Verification items for the finished model (mm, model axes). Face numbers are marked on the shaded views. Coordinates: 2 decimals unless noted, no trailing zeros. Loops run counter-clockwise (first coordinate to the right, second up) from the corner with the lowest first, then second, coordinate; pieces in that order, holes last.
Q1. Material ranges on probe 1 along X at (y, z) = (12.5, -59.69); probe 2 along Z at (x, y) = (-127, 17.5); probe 3 along Z at (x, y) = (-137, 17.5), recorded low to high.
Q2. Sectioned sample at A-A (x = -127). Enter the section's corners in (y, z).
Q3. Mould release check, pull along Z, two halves, no side actions. Record for the marked faces 1, 2 and 3: +Z half, -Z half, draft (parallel to the pull), parting line (faces both ways), or undercut.
Q4. Sectioned sample at D-D (z = -141). Enter the section's corners in (x, y).
Q5. Sectioned sample at C-C (y = 8.5). Enter the section's corners in (x, z), then the cut area to 3 significant figures.
Q6. Go/stop test with flat-tipped pins: P1, Ø1, axis at x = -216, y = 13.5, coming from the -Z side; P2, Ø1, axis at y = 13, z = -130.5, coming from the +X side; P3, Ø8, axis at x = -60.5, y = 13.5, coming from the +Z side. Record where each tip stops, or that it passes through.
Q7. Sectioned sample at B-B (z = -59.69). Enter the section's corners in (x, y), then the cut area to 3 significant figures.
Autodesk Inventor part; units mm, degrees
ref_plane "YZ Plane" through (0, 0, 0) normal (1, 0, 0) x (0, 1, 0)
ref_plane "XZ Plane" through (0, 0, 0) normal (0, 1, 0) x (-1, 0, 0)
ref_plane "XY Plane" through (0, 0, 0) normal (0, 0, 1) x (1, 0, 0)
sketch "Sketch1" plane through (0, 0, 0) normal (0, 1, 0) x (-1, 0, 0)
  line L0 (0, 0) -> (254, 0)
  line L1 (254, 0) -> (254, -119.38)
  line L2 (254, -119.38) -> (0, -119.38)
  line L3 (0, -119.38) -> (0, 0)
  line L4 (186.69, 67.31) -> (67.31, 67.31)
  line L5 (67.31, 67.31) -> (67.31, -186.69)
  line L6 (67.31, -186.69) -> (186.69, -186.69)
  line L7 (186.69, -186.69) -> (186.69, 67.31)
  line L8 (186.69, 67.31) -> (254, 0)
  line L9 (67.31, 67.31) -> (0, 0)
  line L10 (186.69, -186.69) -> (254, -119.38)
  line L11 (0, -119.38) -> (67.31, -186.69)
  line L12 (62.2907, -7.1202) -> (161.0967, -7.1202)
  line L13 (164.2717, -10.2952) -> (164.2717, -109.1012)
  line L14 (161.0967, -112.2762) -> (62.2907, -112.2762)
  line L15 (59.1157, -109.1012) -> (59.1157, -10.2952)
  arc A0 (62.2907, -7.1202) -> (59.1157, -10.2952) centre (62.2907, -10.2952) ccw
  arc A1 (164.2717, -10.2952) -> (161.0967, -7.1202) centre (161.0967, -10.2952) ccw
  arc A2 (161.0967, -112.2762) -> (164.2717, -109.1012) centre (161.0967, -109.1012) ccw
  arc A3 (59.1157, -109.1012) -> (62.2907, -112.2762) centre (62.2907, -109.1012) ccw
  point P0 (164.2717, -112.2762)
  point P1 (164.2717, -7.1202)
  point P2 (59.1157, -112.2762)
  dimension "d0" = 254
  dimension "d1" = 119.38
  dimension "d2" = 119.38
  dimension "d3" = 254
  dimension "d8" = 95.1907
  dimension "d14" = 105.156
  dimension "d15" = 105.156
  dimension "d22" = 3.175
extrude "Extrusion1" add sketch "Sketch1" along normal blind 25.4
sketch "Sketch4" plane through (0, 25.4, 0) normal (0, 1, 0) x (1, 0, 0)
  circle A0 centre (-127, 59.69) radius 25.4
  line L0 (-254, 59.69) -> (-127, 59.69)
  line L1 (-127, 59.69) -> (-127, 186.69)
  line L2 (-254, 119.38) -> (-254, 0)
  line L3 (-67.31, 186.69) -> (-186.69, 186.69)
  point P0 (0, 0)
  dimension "d50" = 50.8
  dimension "d58" = 127
  dimension "d59" = 127
extrude "Extrusion3" cut sketch "Sketch4" against normal blind 25.4
equation "\"d0\" = rectangle_L"
equation "\"d1\" = rectangle_01_w"
equation "\"d2\" = rectangle_01_w"
equation "\"d3\" = rectangle_L"
equation "\"d8\" = d9"
equation "\"rectangle_L\" = 254"
equation "\"rectangle_01_w\" = 119.38"
equation "\"d9\" = 95.19071"
equation "\"window_L\" = 105.156"
equation "\"test\" = 74.422"
equation "\"electrode_diam\" = 50.8"
equation "\"test_points\" = 127"
properties part number "chamber_base"
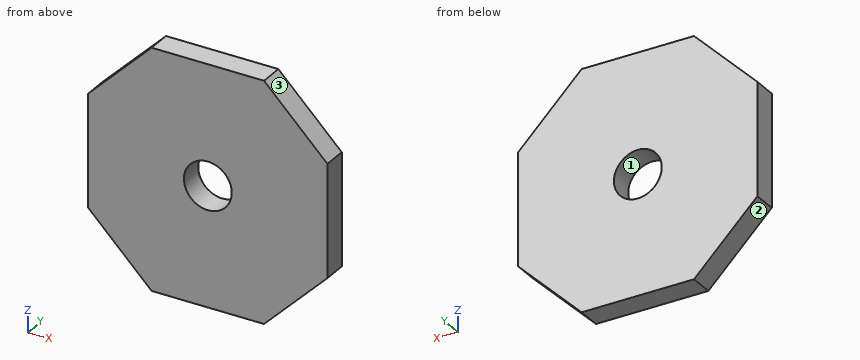
Geometry check:
1. probe 1: x = -254 to -152.4, -101.6 to 0
1. probe 2: z = -186.69 to -85.09, -34.29 to 67.31
1. probe 3: z = -186.69 to -83.04, -36.34 to 67.31
2. outline: (0, -186.69) - (25.4, -186.69) - (25.4, -85.09) - (0, -85.09) - close; (0, -34.29) - (25.4, -34.29) - (25.4, 67.31) - (0, 67.31) - close
3. face 1: undercut
3. face 2: -Z half
3. face 3: +Z half
4. outline: (-232.38, 0) - (-21.62, 0) - (-21.62, 25.4) - (-232.38, 25.4) - close
5. outline: (-254, -119.38) - (-186.69, -186.69) - (-67.31, -186.69) - (0, -119.38) - (0, 0) - (-67.31, 67.31) - (-186.69, 67.31) - (-254, 0) - close; hole circle Ø50.8 at (-127, -59.69)
5. area: 53,400 mm2
6. P1: stops at z = -157.88
6. P2: stops at x = -10.62
6. P3: stops at z = 64.5
7. outline: (-254, 0) - (-152.4, 0) - (-152.4, 25.4) - (-254, 25.4) - close; (-101.6, 0) - (0, 0) - (0, 25.4) - (-101.6, 25.4) - close
7. area: 5,160 mm2
